Build history of the part. All positions in model axes, mm. Face numbers are marked on the shaded views. A direction names the side the tool comes from. Give positions to 0.01 mm unless a question says otherwise; leave off trailing zeros. Write each loop counter-clockwise with the first axis right and the second up, starting at its lowest first coordinate (ties: lowest second). Pieces come first, ordered by that corner, then holes. Notation, with made-up numbers: (25.5, -28.75) - (31.5, -28.75) arc R25 cw to (31.5, -15.75) - close; hole circle Ø6 at (-15, 83.25). An arc over 180 degrees is marked (long way). Use one line per item in the form item = value. Start each with the question number.
Autodesk Inventor part; units mm, degrees
ref_plane "YZ Plane" through (0, 0, 0) normal (1, 0, 0) x (0, 1, 0)
ref_plane "XZ Plane" through (0, 0, 0) normal (0, 1, 0) x (-1, 0, 0)
ref_plane "XY Plane" through (0, 0, 0) normal (0, 0, 1) x (1, 0, 0)
sketch "Sketch1" plane through (0, 0, 0) normal (0, 0, 1) x (1, 0, 0)
  line L0 (-9.9011, 30.8282) -> (2.0989, 30.8282)
  line L1 (2.0989, 30.8282) -> (2.0989, -19.1718)
  line L2 (2.0989, -19.1718) -> (-9.9011, -19.1718)
  line L3 (-9.9011, -19.1718) -> (-9.9011, 30.8282)
  point P0 (0, 0)
  dimension "d0" = 50
  dimension "d1" = 12
extrude "Extrusion1" add sketch "Sketch1" along normal blind 3
sketch "Sketch2" plane through (0, 0, 0) normal (0, 0, -1) x (-1, 0, 0)
  line L0 (-2.0989, -19.1718) -> (-2.0989, 30.8282)
  line L1 (9.9011, -19.1718) -> (-2.0989, -19.1718)
  line L2 (-2.0989, -11.1718) -> (9.9011, -11.1718)
  line L3 (9.9011, -11.1718) -> (9.9011, -19.1718)
  line L4 (9.9011, -19.1718) -> (-2.0989, -19.1718)
  line L5 (-2.0989, -19.1718) -> (-2.0989, -11.1718)
  line L6 (-1.0989, -12.1718) -> (8.9011, -12.1718)
  line L7 (8.9011, -12.1718) -> (8.9011, -18.1718)
  line L8 (8.9011, -18.1718) -> (-1.0989, -18.1718)
  line L9 (-1.0989, -18.1718) -> (-1.0989, -12.1718)
  point P0 (0, 0)
  dimension "d4" = 8
  dimension "d5" = 10
  dimension "d6" = 6
  dimension "d7" = 1
  dimension "d8" = 1
  dimension "d9" = 12
extrude "Extrusion2" cut sketch "Sketch2" against normal blind 1 contours L6 L7 L8 L9
sketch "Sketch3" plane through (0, 0, 0) normal (0, 0, -1) x (-1, 0, 0)
  line L0 (-2.0989, -19.1718) -> (-2.0989, 30.8282)
  line L1 (-2.0989, 30.8282) -> (9.9011, 30.8282)
  line L2 (9.9011, 30.8282) -> (9.9011, -19.1718)
  circle A0 centre (3.9011, 24.8282) radius 2.5
  line L3 (-2.0989, 30.8282) -> (9.9011, 30.8282)
  line L4 (9.9011, 30.8282) -> (9.9011, 18.8282)
  line L5 (9.9011, 18.8282) -> (-2.0989, 18.8282)
  line L6 (-2.0989, 18.8282) -> (-2.0989, 30.8282)
  point P0 (0, 0)
  dimension "d12" = 5
  dimension "d13" = 6
  dimension "d14" = 12
  dimension "d15" = 12
  dimension "d16" = 6
extrude "Extrusion3" add sketch "Sketch3" along normal blind 5 contours A0
fillet "Fillet1" radius 1 1 edges at (-1.4011, 24.8282, 0)
sketch "Sketch4" plane through (0, 0, 3) normal (0, 0, 1) x (1, 0, 0)
  line L0 (2.0989, -19.1718) -> (2.0989, 30.8282)
  line L1 (-9.9011, 5.8282) -> (2.0989, 5.8282)
  line L2 (2.0989, 5.8282) -> (2.0989, -9.1718)
  line L3 (2.0989, -9.1718) -> (-9.9011, -9.1718)
  line L4 (-9.9011, -9.1718) -> (-9.9011, 5.8282)
  line L5 (-9.9011, 30.8282) -> (-9.9011, -19.1718)
  line L6 (-9.9011, -19.1718) -> (2.0989, -19.1718)
  line L7 (2.0989, -19.1718) -> (2.0989, 30.8282)
  line L8 (2.0989, 30.8282) -> (-9.9011, 30.8282)
  line L9 (-9.9011, 30.8282) -> (-9.9011, -19.1718)
  point P0 (0, 0)
  point P1 (2.0989, 5.8282)
  dimension "d20" = 15
  dimension "d21" = 10
extrude "Extrusion4" add sketch "Sketch4" along normal blind 3 contours L3 L4 L1 L0
sketch "Sketch5" plane through (0, 0, 6) normal (0, 0, 1) x (1, 0, 0)
  line L0 (-5.9011, 3.8282) -> (-1.9011, 3.8282)
  line L1 (-1.9011, 3.8282) -> (-1.9011, -7.1718)
  line L2 (-1.9011, -7.1718) -> (-5.9011, -7.1718)
  line L3 (-5.9011, -7.1718) -> (-5.9011, 3.8282)
  line L4 (-9.9011, -9.1718) -> (2.0989, -9.1718)
  line L5 (2.0989, -9.1718) -> (2.0989, 5.8282)
  line L6 (2.0989, 5.8282) -> (-9.9011, 5.8282)
  line L7 (-9.9011, 5.8282) -> (-9.9011, -9.1718)
  point P0 (0, 0)
  dimension "d24" = 12
  dimension "d25" = 15
  dimension "d26" = 4
  dimension "d27" = 11
  dimension "d28" = 4
  dimension "d29" = 2
extrude "Extrusion5" add sketch "Sketch5" along normal blind 5 contours L0 L1 L2 L3
fillet "Fillet2" radius 5 2 edges at (-9.9011, 30.8282, 1.5) (2.0989, 30.8282, 1.5)
sketch "Sketch6" plane through (0, 0, 3) normal (0, 0, 1) x (1, 0, 0)
  circle A0 centre (-3.9011, 24.8282) radius 2.5
  line L0 (-6.4011, 24.8282) -> (-1.4011, 24.8282)
  line L1 (-1.4011, 24.8282) -> (-1.4011, 5.8282)
  line L2 (-1.4011, 5.8282) -> (-6.4011, 5.8282)
  line L3 (-6.4011, 5.8282) -> (-6.4011, 24.8282)
  line L4 (2.0989, 5.8282) -> (-9.9011, 5.8282)
  line L5 (2.0989, -9.1718) -> (-9.9011, -9.1718)
  line L6 (-6.4011, -9.1718) -> (-1.4011, -9.1718)
  line L7 (-1.4011, -9.1718) -> (-1.4011, -19.1718)
  line L8 (-1.4011, -19.1718) -> (-6.4011, -19.1718)
  line L9 (-6.4011, -19.1718) -> (-6.4011, -9.1718)
  line L10 (-9.9011, -19.1718) -> (2.0989, -19.1718)
  point P0 (0, 0)
  point P1 (-1.4011, -9.1718)
  dimension "d38" = 5
  dimension "d39" = 5
extrude "Extrusion6" add sketch "Sketch6" along normal blind 1.5
chamfer "Chamfer1" distance 1.5 angle 45 6 edges at (-1.4011, 15.3282, 3) (-3.9011, 27.3282, 3) (-6.4011, 15.3282, 3) (-6.4011, -14.1718, 3) (-1.4011, -14.1718, 3) (-3.9011, -19.1718, 4.5)
equation "\"d7\" = -0.5 * d5 + 0.5 * d9"
equation "\"d8\" = -0.5 * d6 + 0.5 * d4"
equation "\"d13\" = 0.5 * d14"
equation "\"d15\" = d14"
equation "\"d16\" = 0.5 * d14"
equation "\"d26\" = 0.333333 * d24"
equation "\"d28\" = -0.5 * d26 + 0.5 * d24"
equation "\"d39\" = d38"
properties part number "wheel connector"
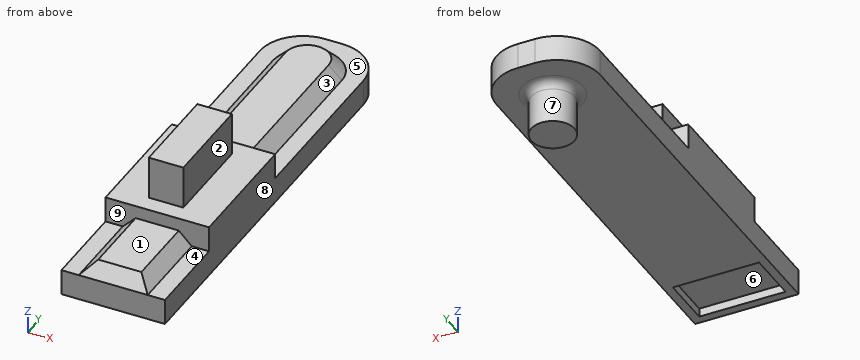
(1) Wall check: line 1 (Y direction, x = 0.75, z = 4.75); line 2 (Z direction, x = 1.5, y = 17.5); line 3 (Z direction, x = -4.75, y = 27). Give the ranges that are in metal, low to high. Write a range as from..to.
(2) Which spindle directions (+Z, -Z, +X, -X, +Y, -Y) get a long thin tool onto all of the face, cutting with end or side? Do the marked faces 1, 2, 3, 4 and 5. Say none if no direction does.
(3) Cut at B-B, the plane z = 2.25. Give the cut face in (x, y), then the cut area to 3 significant figures.
(4) Cut at C-C, the plane y = 0.5. Give the cut face in (x, z).
(5) Pin check, flat tips, straight feed: pin 1 Ø3.5 at (x, y) = (-2, 3) entering from -Z; pin 2 Ø1.5 at (y, z) = (3.5, 8.5) entering from -X; pin 3 Ø5.5 at (y, z) = (-3, 8.5) entering from +X; pin 4 Ø2.5 at (x, y) = (-3, -13) entering from +Z. Stop position of each tip, or through.
(6) Two-plate mould, pull along Y, no slides. Class the marked faces 6, 7, 8 and 9: +Y half, -Y half, draft (parallel to the pull), parting line (faces both ways), or undercut.
(7) Cut at D-D, the plane z = -3. Give the cut face in (x, y).
Solution:
q1.line_1 = -9.17..5.83
q1.line_2 = 0..3
q1.line_3 = -5..4.5
q2.face_1 = +Z, +X, -X, -Y
q2.face_2 = +Z, +X, +Y, -Y
q2.face_3 = +Z, +X, +Y
q2.face_4 = +Z, +X, -Y
q2.face_5 = +Z, +Y
q3.outline = (-9.9, -19.17) - (2.1, -19.17) - (2.1, 25.83) arc R5 ccw to (-2.9, 30.83) - (-4.9, 30.83) arc R5 ccw to (-9.9, 25.83) - close
q3.area = 589 mm2
q4.outline = (-9.9, 0) - (2.1, 0) - (2.1, 6) - (-1.9, 6) - (-1.9, 11) - (-5.9, 11) - (-5.9, 6) - (-9.9, 6) - close
q5.pin_1 = 0
q5.pin_2 = -5.9
q5.pin_3 = 2.1
q5.pin_4 = 4.5
q6.face_6 = undercut
q6.face_7 = parting line
q6.face_8 = draft
q6.face_9 = -Y half
q7.outline = circle Ø5 at (-3.9, 24.83)
